from build123d import *

# Parameters (mm, degrees)
SKETCH1_W           = 74.2
SKETCH1_H           = 11.2
SKETCH1_W_2         = 68.2
SKETCH1_H_2         = 5.2
BOSS_EXTRUDE1_DEPTH = 1.7
SKETCH2_W           = 74.2
SKETCH2_H           = 11.2
BOSS_EXTRUDE2_DEPTH = 3
SKETCH5_R           = 1
CUT_EXTRUDE1_DEPTH  = 3
CUT_EXTRUDE2_DEPTH  = 1.6
SKETCH8_W           = 27.1
SKETCH8_H           = 5.2
BOSS_EXTRUDE3_DEPTH = 1.7


with BuildPart() as part:
    # Sketch1 → Boss-Extrude1 (new body)
    with BuildSketch(Plane(origin=(0, 0, 0), x_dir=(1, 0, 0), z_dir=(0, 1, 0))):
        Rectangle(SKETCH1_W, SKETCH1_H)
        Rectangle(SKETCH1_W_2, SKETCH1_H_2, mode=Mode.SUBTRACT)
    extrude(amount=-BOSS_EXTRUDE1_DEPTH)

    # Sketch2 → Boss-Extrude2 (add)
    with BuildSketch(Plane.XZ.offset(1.7)):
        Rectangle(SKETCH2_W, SKETCH2_H)
    extrude(amount=BOSS_EXTRUDE2_DEPTH)

    # Sketch5 → Cut-Extrude1 (cut)
    with BuildSketch(Plane(origin=(0, -1.7, 0), x_dir=(1, 0, 0), z_dir=(0, 1, 0))):
        with Locations(Location((-4, 0, 0), (0, 0, 270))):
            Circle(SKETCH5_R)
        with Locations(Location((31, 0, 0), (0, 0, 270))):
            Circle(SKETCH5_R)
    extrude(amount=-CUT_EXTRUDE1_DEPTH, mode=Mode.SUBTRACT)

    # Sketch7 → Cut-Extrude2 (cut)
    with BuildSketch(Plane.XZ.offset(4.7)):
        Polygon((-5.15, 1.991858429), (-6.3, 0), (-5.15, -1.991858429), (-2.85, -1.991858429), (-1.7, 0), (-2.85, 1.991858429), align=None)
        Polygon((33.3, 0), (32.15, 1.991858429), (29.85, 1.991858429), (28.7, 0), (29.85, -1.991858429), (32.15, -1.991858429), align=None)
    extrude(amount=-CUT_EXTRUDE2_DEPTH, mode=Mode.SUBTRACT)

    # Sketch8 → Boss-Extrude3 (add)
    with BuildSketch(Plane(origin=(0, -1.7, 0), x_dir=(1, 0, 0), z_dir=(0, 1, 0))):
        with Locations((-20.55, 0)):
            Rectangle(SKETCH8_W, SKETCH8_H)
    extrude(amount=BOSS_EXTRUDE3_DEPTH)


solid = part.part
The model under review builds one solid part; all positions refer to its coordinate system, in mm. A direction names the side the tool comes from. Coordinates: 2 decimals unless noted, no trailing zeros. Write each loop counter-clockwise with the first axis right and the second up, starting at its lowest first coordinate (ties: lowest second). Pieces come first, ordered by that corner, then holes. Notation, with made-up numbers: M -4.5,5 L 41.5,5 A35 ccw 41.5,44 Z; hole C 33.5,-17 d4. An arc over 180 degrees is marked long. Put each result on its own line as item: value.
1) Wall thickness on probe 1 along X at (y, z) = (-2.25, 0); probe 2 along X at (y, z) = (-4, 1.75); probe 3 along Y at (x, z) = (11, -1.75): over which ranges is each line inside the solid? List them lowest first. Write a range as [from, to].
Computed:
probe 1: x = [-37.1, -5], [-3, 30], [32, 37.1]
probe 2: x = [-37.1, -5.29], [-2.71, 29.71], [32.29, 37.1]
probe 3: y = [-4.7, -1.7]
2) Draft analysis for pull direction Z (two halves, no side actions). For faces 1 (the flat face through (-1, -4.7, 0)), 2 (the flat face through (-1, -2, 5.6)), 3 (the flat face through (-5, -3.1, 1)), 4 (the flat face through (29.283, -3.911, 1.01)), state which applies: released by +Z, released by -Z, zero draft, split by the parting line, or undercut.
Computed:
face 1: zero draft
face 2: released by +Z
face 3: undercut
face 4: undercut
3) Add section A-A on y = -3.95. Give the boundary of the cut face in (x, z), then the cut area to 3 significant figures.
Computed:
outline: M -37.1,-5.6 L 37.1,-5.6 L 37.1,5.6 L -37.1,5.6 Z; hole M -6.3,0 L -5.15,-1.99 L -2.85,-1.99 L -1.7,0 L -2.85,1.99 L -5.15,1.99 Z; hole M 28.7,0 L 29.85,-1.99 L 32.15,-1.99 L 33.3,0 L 32.15,1.99 L 29.85,1.99 Z
area: 804 mm2
4) Clearance check with flat-ended pins moving along their axes: pin 1 Ø1.6 at (x, z) = (4, 0.5) entering from +Y; pin 2 Ø1.2 at (x, z) = (-4, -0.5) entering from -Y. State where each tip first meets the part, or that it passes through.
Computed:
pin 1: stops at y = -1.7
pin 2: stops at y = -3.1
5) Add section B-B on x = -4. Give the boundary of the cut face in (y, z), then the cut area to 3 significant figures.
Computed:
outline: M -4.7,-5.6 L 0,-5.6 L 0,-2.6 L -1.7,-2.6 L -1.7,-1 L -3.1,-1 L -3.1,-1.99 L -4.7,-1.99 Z; M -4.7,1.99 L -3.1,1.99 L -3.1,1 L -1.7,1 L -1.7,2.6 L 0,2.6 L 0,5.6 L -4.7,5.6 Z
area: 34.6 mm2
6) For faces 5 (the flat face through (31, -4, -1.992)), 6 (the flat face through (37.1, -2, 0)), 7 (the flat face through (34.1, -1, 0)), list the 3-axis set-ups (+Z, -Z, +X, -X, +Y, -Y) from which the entire face can be reached by the end or side of a thin tool; tool diameter is ignored.
Computed:
face 5: -Y
face 6: +Z, -Z, +X, +Y, -Y
face 7: +Y
